The listing builds one solid part. Answer for the finished solid, in the listing's coordinates (mm). A direction names the side the tool comes from. Coordinates: 2 decimals unless noted, no trailing zeros. Order: outer loops, then holes, each group sorted by start corner. A loop starts at its lowest first (then second) coordinate and runs counter-clockwise, first axis right, second up. Notation, with made-up numbers: (84, 79) - (131, 79) arc R22 cw to (131, 97) - close; hole circle Ø4 at (-24, 19.25). An arc over 180 degrees is marked (long way). Use a Markdown table: item, result. Add a question column.
Item 1: The mould has two halves that part along Z. Classify faces 1 (the flat face through (33.056, 0.986, 12.773)), 2 (the flat face through (-6, 2, 2)): released by +Z, released by -Z, zero draft, split by the parting line, or undercut.
Item 2: The part is cut by section C-C, the plane x = -21. Give the vertices of the cut face in (y, z).
Item 3: For faces 3 (the flat face through (-6, 0, 2)), 4 (the flat face through (35.15, 0.99, 1.32)), determine the directions among +Z, -Z, +X, -X, +Y, -Y from which every point of the face is accessible in a straight line to the end or side of a thin tool.
Item 4: The part is cut by section D-D, the plane z = 8. Give the vertices of the cut face in (x, y), then the cut area to 3 significant figures.
Item 5: Find the intervals of material crossed by line 1 along Z through (x, y) = (-69, 1.35); line 2 along X through (y, z) = (1.25, 23.5); line 3 along Z through (x, y) = (-14, 1.4), in increasing order.
Item 6: Flat-ended cylindrical pins translate along their axes: P1, Ø0.6, axis at x = -21.5, y = 1, coming from the -Z side; P2, Ø0.6, axis at y = 1, z = -12.5, coming from the +X side. Find the tip coordinate at first contact, or state that the pin passes through.
Item 7: The part is cut by section B-B, the plane x = 62. Give the vertices of the cut face in (y, z), then the cut area to 3 significant figures.
from build123d import *

# Parameters (mm, degrees)
BOSS_EXTRUDE1_DEPTH = 2
FILLET1_R           = 1
FILLET2_R           = 2
FILLET3_R           = 2.5


with BuildPart() as part:
    # Sketch1 → Boss-Extrude1 (new body)
    with BuildSketch(Plane(origin=(0, 0, 0), x_dir=(1, 0, 0), z_dir=(0, 1, 0))):
        with BuildLine():
            ThreePointArc((-40.844914922, -4.388665388), (-43.544914922, -7.088665388), (-40.844914922, -9.788665388))
            Line((-40.844914922, -9.788665388), (111.455085078, -15.938665388))
            Line((111.455085078, -15.938665388), (111.455085078, -22.938665388))
            Line((111.455085078, -22.938665388), (-69.544914922, -22.938665388))
            Line((-69.544914922, -22.938665388), (-74.131846847, -22.938665388))
            ThreePointArc((-74.131846847, -22.938665388), (-77.344914922, -23.713665388), (-74.131846847, -24.488665388))
            Line((-74.131846847, -24.488665388), (-69.544914922, -24.488665388))
            Line((-69.544914922, -24.488665388), (-69.544914922, -29.288665388))
            Line((-69.544914922, -29.288665388), (-83.544914922, -29.288665388))
            Line((-83.544914922, -29.288665388), (-83.544914922, 15.111334612))
            Line((-83.544914922, 15.111334612), (-69.544914922, 15.111334612))
            Line((-69.544914922, 15.111334612), (-69.544914922, 10.311334612))
            Line((-69.544914922, 10.311334612), (-74.131846847, 10.311334612))
            ThreePointArc((-74.131846847, 10.311334612), (-77.344914922, 9.536334612), (-74.131846847, 8.761334612))
            Line((-74.131846847, 8.761334612), (-69.544914922, 8.761334612))
            Line((-69.544914922, 8.761334612), (111.455085078, 8.761334612))
            Line((111.455085078, 8.761334612), (111.455085078, 1.761334612))
            Line((111.455085078, 1.761334612), (-40.844914922, -4.388665388))
        make_face()
    extrude(amount=BOSS_EXTRUDE1_DEPTH)

    # Fillet1
    fillet1_edges = [part.edges().sort_by_distance(p)[0] for p in [
        (-74.131846847, 1, 22.938665388),
        (-74.131846847, 1, 24.488665388),
        (-83.544914922, 1, 29.288665388),
        (-83.544914922, 1, -15.111334612),
        (-74.131846847, 1, -10.311334612),
        (-74.131846847, 1, -8.761334612),
    ]]
    fillet(fillet1_edges, radius=FILLET1_R)

    # Fillet2
    fillet2_edges = [part.edges().sort_by_distance(p)[0] for p in [
        (-69.544914922, 1, 24.488665388),
        (-69.544914922, 1, 29.288665388),
        (-69.544914922, 1, -15.111334612),
        (-69.544914922, 1, -10.311334612),
    ]]
    fillet(fillet2_edges, radius=FILLET2_R)

    # Fillet3
    fillet3_edges = [part.edges().sort_by_distance(p)[0] for p in [
        (111.455085078, 1, 15.938665388),
        (111.455085078, 1, 22.938665388),
        (111.455085078, 1, -8.761334612),
        (111.455085078, 1, -1.761334612),
    ]]
    fillet(fillet3_edges, radius=FILLET3_R)


solid = part.part
Solution:
| question | item | result |
|---|---|---|
| 1 | face 1 | undercut |
| 1 | face 2 | zero draft |
| 2 | outline | (0, -8.76) - (2, -8.76) - (2, 3.59) - (0, 3.59) - close; (0, 10.59) - (2, 10.59) - (2, 22.94) - (0, 22.94) - close |
| 3 | face 3 | +Z, -Z, +X, -X, -Y |
| 3 | face 4 | +X, +Y, -Y |
| 4 | outline | (-83.54, 0) - (-43.39, 0) - (-43.39, 2) - (-83.54, 2) - close |
| 4 | area | 80.3 mm2 |
| 5 | line 1 | z = -8.76 to 22.94 |
| 5 | line 2 | x = -83.54 to -77.33 |
| 5 | line 3 | z = -8.76 to 3.3, 10.87 to 22.94 |
| 6 | P1 | stops at z = -8.76 |
| 6 | P2 | stops at x = -69.54 |
| 7 | outline | (0, -8.76) - (2, -8.76) - (2, 0.24) - (0, 0.24) - close; (0, 13.94) - (2, 13.94) - (2, 22.94) - (0, 22.94) - close |
| 7 | area | 36.0 mm2 |
